For this review, take the finished solid that the model builds, in its own axes (mm). A direction names the side the tool comes from. Round coordinates to 2 decimals unless told otherwise and drop trailing zeros. Write each loop counter-clockwise with the first axis right and the second up, starting at its lowest first coordinate (ties: lowest second). Pieces come first, ordered by that corner, then holes. Notation, with made-up numbers: (88, 39.25) -> (132, 39.25) arc R26 ccw to (132, 56.25) -> close; hole circle Ø2 at (87, 61). An arc over 180 degrees is marked (long way). Answer in a Markdown table with one row per item.
from build123d import *

# Parameters (mm, degrees)
SKETCH_1_R               = 22.5
EXTRUDE_2_DEPTH          = 3.2
PATTERN_CIRCULAR_2_COUNT = 15
SKETCH_3_R               = 3.25
CUT_EXTRUDE_2_DEPTH      = 3.2
SKETCH_5_R               = 1.6
CUT_EXTRUDE_3_DEPTH      = 10


with BuildPart() as part:
    # ｽｹｯﾁ1 → ﾎﾞｽ - 押し出し2 (new body)
    with BuildSketch(Plane.XY):
        Circle(SKETCH_1_R)
        with BuildLine():
            Line((0, 0), (-2.5, 0))
            Line((-2.5, 0), (-2.5, 40))
            Line((-2.5, 40), (-6.5, 40))
            Line((-6.5, 40), (-6.5, 43.517237964))
            ThreePointArc((-6.5, 43.517237964), (-0.454315658, 43.997654452), (5.6, 43.64218143))
            Line((5.6, 43.64218143), (5.6, 40))
            Line((5.6, 40), (2.5, 40))
            Line((2.5, 40), (2.5, 0))
            Line((2.5, 0), (0, 0))
        make_face()
    extrude_2 = extrude(amount=EXTRUDE_2_DEPTH)

    # 円形ﾊﾟﾀｰﾝ2: ﾎﾞｽ - 押し出し2 ×15 about axis
    pattern_circular_2_axis = Axis((0, 0, 0), (0, 0, 1))
    for i in range(1, PATTERN_CIRCULAR_2_COUNT):
        add(extrude_2.rotate(pattern_circular_2_axis, i * 360 / PATTERN_CIRCULAR_2_COUNT))

    # ｽｹｯﾁ3 → ｶｯﾄ - 押し出し2 (cut)
    with BuildSketch(Plane.XY.offset(3.2)):
        Circle(SKETCH_3_R)
    extrude(amount=-CUT_EXTRUDE_2_DEPTH, mode=Mode.SUBTRACT)

    # ｽｹｯﾁ5 → ｶｯﾄ - 押し出し3 (cut)
    with BuildSketch(Plane.XY.offset(3.2)):
        with Locations((-15, 0)):
            Circle(SKETCH_5_R)
        with Locations((15, 0)):
            Circle(SKETCH_5_R)
    extrude(amount=-CUT_EXTRUDE_3_DEPTH, mode=Mode.SUBTRACT)


solid = part.part
1) Consider section B-B on z = 1.35. State how many separate pieces and enclosed holes the cut face has, then the cut area to 3 significant figures.
Solved:
| item | result |
|---|---|
| separate pieces | 1 |
| enclosed holes | 3 |
| area | 3,560 mm² |
2) Consider section A-A on x = 0. State the section outline as (y, z) points.
Solved:
| item | result |
|---|---|
| outline | (-22.5, 0) -> (-3.25, 0) -> (-3.25, 3.2) -> (-22.5, 3.2) -> close; (3.25, 0) -> (44, 0) -> (44, 3.2) -> (3.25, 3.2) -> close |
3) For faces 3 (the flat face through (34.8, 23.8, 1.6)), 4 (the cylindrical face through (19.501, 11.223, 1.578)), 5 (the flat face through (-42.203, 1.195, 1.578)), list the 3-axis set-ups (+Z, -Z, +X, -X, +Y, -Y) from which the entire face can be reached by the end or side of a thin tool; tool diameter is ignored.
Solved:
| item | result |
|---|---|
| face 3 | +Z, -Z, +X |
| face 4 | +Z, -Z |
| face 5 | +Z, -Z, -X |
4) Mouldability with a two-part tool opening along Y and no side actions: class faces 1 (the flat face through (-2.32, -42.17, 1.58)), 2 (the flat face through (27.13, -29.73, 1.58)) as pulls with the +Y half, pulls with the -Y half, needs draft (parallel to the pull), parting line crosses it, or undercut.
Solved:
| item | result |
|---|---|
| face 1 | pulls with the -Y half |
| face 2 | undercut |
5) For line 1 (Y direction, x = 0, z = 2.6); line 2 (Y direction, x = -24.5, z = 0.7); line 3 (Y direction, x = -29, z = 1.2), list the stretches that pass through material, from the lowest coordinate up. Write a range as [from, to].
Solved:
| item | result |
|---|---|
| line 1 | [-22.5, -3.25], [3.25, 44] |
| line 2 | [-36.55, -29.47], [-17.03, -11.26], [-5.09, -0.06], [5.33, 10.59], [18.7, 25.42] |
| line 3 | [-33.09, -30.39], [-19.63, -13.86], [-5.56, -0.53], [6.79, 12.05], [22.75, 33.09] |
6) Clearance check with flat-ended pins moving along their axes: pin 1 Ø1 at (x, z) = (-4.5, 2) entering from -Y; pin 2 Ø1 at (y, z) = (35, 1.5) entering from +X; pin 3 Ø1.6 at (y, z) = (41, 1.5) entering from +X. State where each tip first meets the part, or that it passes through.
Solved:
| item | result |
|---|---|
| pin 1 | y = -43.82 |
| pin 2 | x = 21.94 |
| pin 3 | x = 17.89 |
